Model file for the job. Use its own axes, mm. A direction names the side the tool comes from. Round coordinates to 2 decimals unless told otherwise and drop trailing zeros. Order: outer loops, then holes, each group sorted by start corner. A loop starts at its lowest first (then second) coordinate and runs counter-clockwise, first axis right, second up. Notation, with made-up numbers: (-33, -26) - (-3, -26) arc R28 cw to (-3, 13) - close; hole circle Ø11 at (-28.75, 37). An arc over 180 degrees is marked (long way). Use one line per item in the form item = value.
from build123d import *

# Parameters (mm, degrees)
SKETCH1_R           = 5
BOSS_EXTRUDE1_DEPTH = 5


with BuildPart() as part:
    # Sketch1 → Boss-Extrude1 (new body, symmetric)
    with BuildSketch(Plane(origin=(0, 0, 0), x_dir=(0, 0, -1), z_dir=(1, 0, 0))):
        with BuildLine():
            Line((0, 15), (-20, 15))
            Line((-20, 15), (-20, -15))
            Line((-20, -15), (0, -15))
            ThreePointArc((0, -15), (15, 0), (0, 15))
        make_face()
        Circle(SKETCH1_R, mode=Mode.SUBTRACT)
    extrude(amount=BOSS_EXTRUDE1_DEPTH, both=True)

    # Sketch3 → Revolve1 (revolve)
    with BuildSketch(Plane(origin=(5, 0, 0), x_dir=(0, 0, -1), z_dir=(1, 0, 0))):
        Polygon((-20, 1.817002653), (-20, 15), (-20, 15.485698602), (-20, 18.475930921), (-24, 18.475930921), (-24, 17.713484144), (-244, 17.713484144), (-244, 10.782192935), (-26, 10.782192935), (-26, 0), (-20, 0), align=None)
    revolve(axis=Axis((5, 0, 26), (0, 0, -1)))


solid = part.part
(1) Pull direction Y, two halves, no side cores. Call faces 5 (the face through (-5, 0, 7)), 6 (the face through (-0.07, -4.88, 1.08)), 7 (the face through (0, 0, -15)), 8 (the face through (5, 0, 26)): released by +Y, released by -Y, zero draft, split by the parting line, or undercut.
Report:
face_5 = zero draft
face_6 = undercut
face_7 = split by the parting line
face_8 = undercut
(2) Slice it at C-C on x = -10.5. Give the cut face in (y, z).
Report:
outline = (-10.06, 20) - (10.06, 20) - (10.06, 24) - (8.57, 24) - (8.57, 244) - (-8.57, 244) - (-8.57, 24) - (-10.06, 24) - close
(3) Slice it at B-B on z = 154.5. Give the cut face in (x, y), then the cut area to 4 significant figures.
Report:
outline = circle Ø35.43 at (5, 0); hole circle Ø21.56 at (5, 0)
area = 620.5 mm2
(4) Probe probe 1 along X at (y, z) = (0, 151); probe 2 along Y at (x, z) = (2.25, 0); probe 3 along Z at (x, y) = (0.5, 0.5). List the from-to ranges inside material, lowest first. Write a range as [from, to].
Report:
probe_1 = [-12.71, -5.78], [15.78, 22.71]
probe_2 = [-15, -5], [5, 15]
probe_3 = [-14.99, -4.97], [4.97, 26]
(5) Tool access for faces 1 (the face through (5, 0, 7)), 2 (the face through (0, 15, 10)), 3 (the face through (-13, 1, 24)), 4 (the face through (0, -15, 10)): list every direction of +Z, -Z, +X, -X, +Y, -Y with a clear straight run to the whole face (end or side of a thin tool).
Report:
face_1 = -Z, +X, +Y, -Y
face_2 = -Z, +X, -X, +Y
face_3 = +Z
face_4 = -Z, +X, -X, -Y
(6) Slice it at A-A on y = 0. Give the cut face in (x, z).
Report:
outline = (-13.48, 20) - (-5, 20) - (-5, 5) - (5, 5) - (5, 20) - (23.48, 20) - (23.48, 24) - (22.71, 24) - (22.71, 244) - (15.78, 244) - (15.78, 26) - (-5.78, 26) - (-5.78, 244) - (-12.71, 244) - (-12.71, 24) - (-13.48, 24) - close; (-5, -15) - (5, -15) - (5, -5) - (-5, -5) - close
(7) Slice it at D-D on x = 8.5. Give the cut face in (y, z).
Report:
outline = (-18.14, 20) - (18.14, 20) - (18.14, 24) - (17.36, 24) - (17.36, 244) - (10.2, 244) - (10.2, 26) - (-10.2, 26) - (-10.2, 244) - (-17.36, 244) - (-17.36, 24) - (-18.14, 24) - close
(8) Pin check, flat tips, straight feed: pin 1 (6 mm diameter, centred on y = -11, z = 90.5, fed in from -X); pin 2 (15 mm diameter, centred on y = -3, z = 6, fed in from +X); pin 3 (3 mm diameter, centred on x = -5, z = 35.5, fed in from +Y). Stop position of each tip, or through.
Report:
pin_1 = -10.8
pin_2 = 5
pin_3 = 15.54
